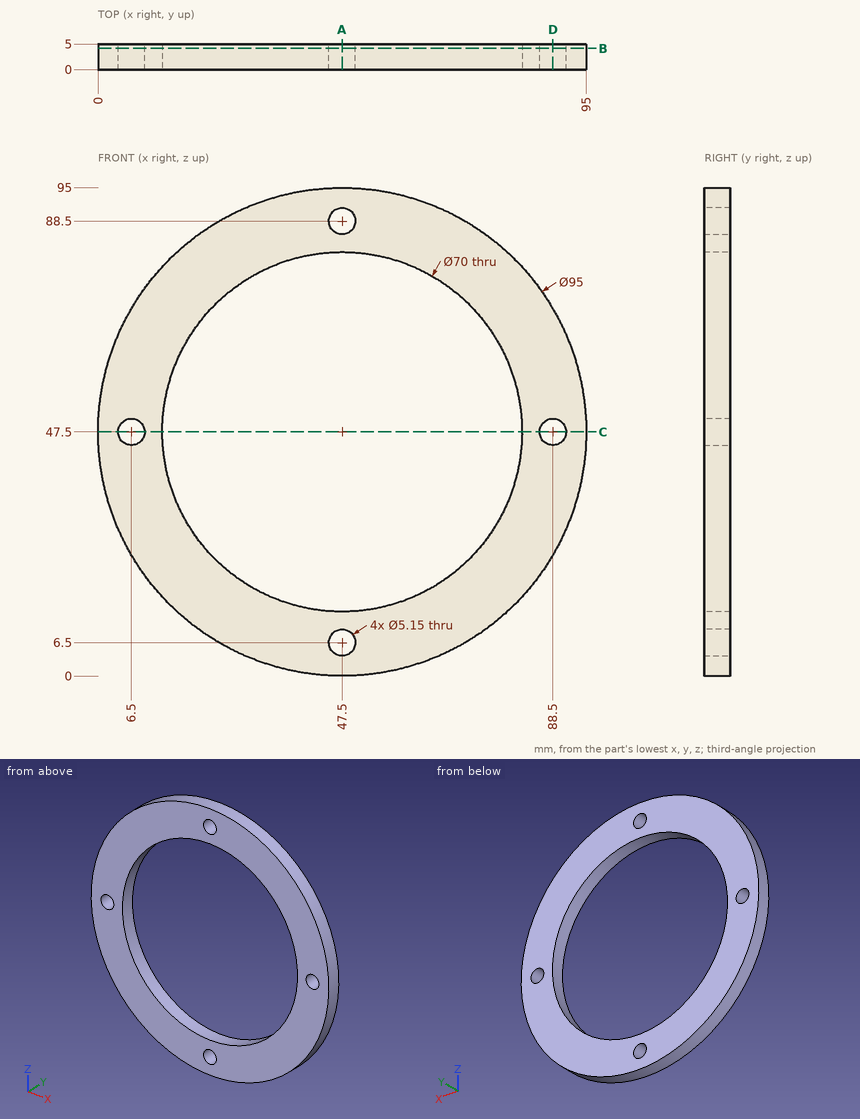
Print and shaded views of the part. All mm, measured from the part's lowest x, y and z. Give positions to 0.01 mm unless a question says otherwise; leave off trailing zeros. Loops run counter-clockwise (first coordinate to the right, second up) from the corner with the lowest first, then second, coordinate; pieces in that order, holes last.
1) Saw through at A-A (x = 47.5). Write the cut outline in (y, z) (3 decimals).
2) Saw through at D-D (x = 88.5). Write the cut outline in (y, z) (3 decimals), plus the area to 3 significant figures.
3) Saw through at B-B (y = 4.15). Write the cut outline in (x, z) (3 decimals), plus the area to 3 significant figures.
4) Flat gauge pin, fed straight in: pin 1 Ø2 at (y, z) = (3, 42) entering from +X. Where does the tip first touch, or does it go through?
5) Wall check: line 1 (X direction, y = 2.15, z = 47.5) (3 decimals); line 2 (Z direction, x = 89.5, y = 3.05); line 3 (X direction, y = 2.95, z = 88.5) (3 decimals). Give the ranges that are in metal, low to high.
6) Saw through at C-C (z = 47.5). Write the cut outline in (x, y) (3 decimals), plus the area to 3 significant figures.
Answer block:
1. outline: (0, 0) - (5, 0) - (5, 3.925) - (0, 3.925) - close; (0, 9.075) - (5, 9.075) - (5, 12.5) - (0, 12.5) - close; (0, 82.5) - (5, 82.5) - (5, 85.925) - (0, 85.925) - close; (0, 91.075) - (5, 91.075) - (5, 95) - (0, 95) - close
2. outline: (0, 23.516) - (5, 23.516) - (5, 44.925) - (0, 44.925) - close; (0, 50.075) - (5, 50.075) - (5, 71.484) - (0, 71.484) - close
2. area: 214 mm2
3. outline: circle Ø95 at (47.5, 47.5); hole circle Ø5.15 at (6.5, 47.5); hole circle Ø70 at (47.5, 47.5); hole circle Ø5.15 at (47.5, 6.5); hole circle Ø5.15 at (47.5, 88.5); hole circle Ø5.15 at (88.5, 47.5)
3. area: 3,160 mm2
4. pin 1: stops at x = 94.79
5. line 1: x = 0 to 3.925, 9.075 to 12.5, 82.5 to 85.925, 91.075 to 95
5. line 2: z = 25.31 to 45.13, 49.87 to 69.69
5. line 3: x = 23.516 to 44.925, 50.075 to 71.484
6. outline: (0, 0) - (3.925, 0) - (3.925, 5) - (0, 5) - close; (9.075, 0) - (12.5, 0) - (12.5, 5) - (9.075, 5) - close; (82.5, 0) - (85.925, 0) - (85.925, 5) - (82.5, 5) - close; (91.075, 0) - (95, 0) - (95, 5) - (91.075, 5) - close
6. area: 73.5 mm2
